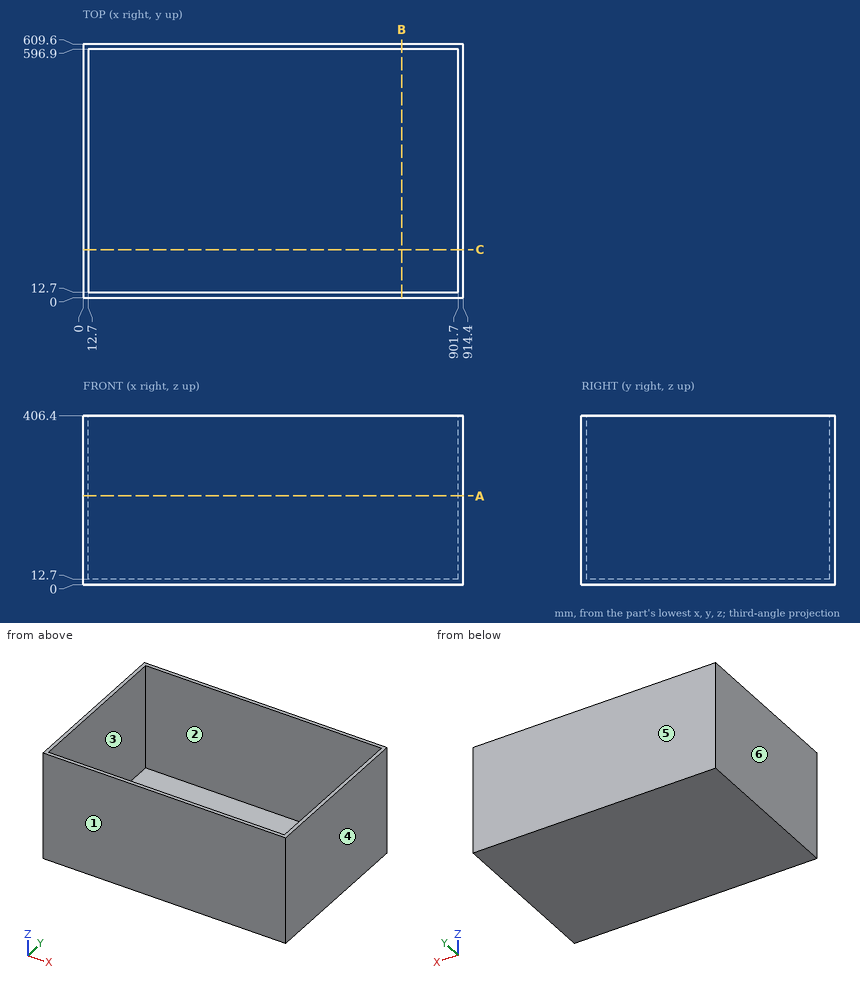
Here's the drawing with two shaded views (mm, measured from the low corner). I have some questions. A direction names the side the tool comes from. Coordinates: 2 decimals unless noted, no trailing zeros. Loops run counter-clockwise (first coordinate to the right, second up) from the corner with the lowest first, then second, coordinate; pieces in that order, holes last. Notation, with made-up numbers: (48, -32) -> (105, -32) arc R21 ccw to (105, 7) -> close; hole circle Ø10 at (78.25, -11.75). An arc over 180 degrees is marked (long way). Answer as a JSON object with one key per item and string values.
1) Imagine slicing it at C-C (y = 115.5). Please give me the cut outline in (x, z), then the cut area to 3 significant figures.
Results:
{"outline": "(0, 0) -> (914.4, 0) -> (914.4, 406.4) -> (901.7, 406.4) -> (901.7, 12.7) -> (12.7, 12.7) -> (12.7, 406.4) -> (0, 406.4) -> close", "area": "21,600 mm^2"}
2) For P1, Ø2, axis at x = 402.5, y = 252, coming from the +Z side; P2, Ø4, axis at x = 621.5, y = 248, coming from the -Z side, each with a flat end and sliding along its axis, tell me the tip position at first contact or that it passes through.
Results:
{"P1": "stops at z = 12.7", "P2": "stops at z = 0"}
3) Imagine slicing it at A-A (z = 213.5). Please give me the cut outline in (x, y).
Results:
{"outline": "(0, 0) -> (914.4, 0) -> (914.4, 609.6) -> (0, 609.6) -> close; hole (12.7, 12.7) -> (901.7, 12.7) -> (901.7, 596.9) -> (12.7, 596.9) -> close"}
4) Imagine slicing it at B-B (x = 766). Please give me the cut outline in (y, z), then the cut area to 3 significant figures.
Results:
{"outline": "(0, 0) -> (609.6, 0) -> (609.6, 406.4) -> (596.9, 406.4) -> (596.9, 12.7) -> (12.7, 12.7) -> (12.7, 406.4) -> (0, 406.4) -> close", "area": "17,700 mm^2"}
5) If I drill on line 1 (Y direction, x = 357, z = 321); line 2 (X direction, y = 581, z = 110); line 3 (Z direction, x = 520.5, y = 319), over which ranges is the centre line in solid material (lowest first)?
Results:
{"line 1": "y = 0 to 12.7, 596.9 to 609.6", "line 2": "x = 0 to 12.7, 901.7 to 914.4", "line 3": "z = 0 to 12.7"}
6) For the marked faces 1 and 2, which set-ups out of +Z, -Z, +X, -X, +Y, -Y let a thin tool reach every point of the face, with its end or its side?
Results:
{"face 1": "+Z, -Z, +X, -X, -Y", "face 2": "+Z"}
7) Thinking about a two-plate mould opening in X: for the marked faces 3, 4, 5 and 6, which applies, pulls with the +X half, pulls with the -X half, needs draft (parallel to the pull), parting line crosses it, or undercut?
Results:
{"face 3": "undercut", "face 4": "pulls with the +X half", "face 5": "needs draft", "face 6": "pulls with the -X half"}
